Here's how the part is built. I have some questions about the finished solid (model axes, mm). Face numbers are marked on the shaded views. A direction names the side the tool comes from. Give positions to 0.01 mm unless a question says otherwise; leave off trailing zeros. Order: outer loops, then holes, each group sorted by start corner. A loop starts at its lowest first (then second) coordinate and runs counter-clockwise, first axis right, second up.
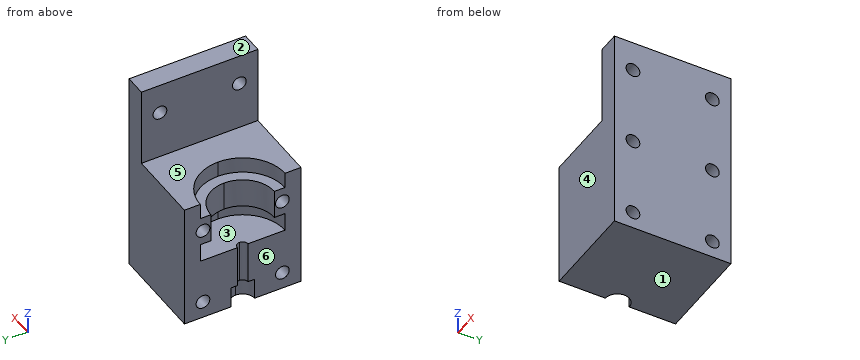
from build123d import *

# Parameters (mm, degrees)
F2_DEPTH  = 24
F1_W      = 3
F1_H      = 22
F3_DEPTH  = 24
F1_W_2    = 4
F4_DEPTH  = 39
F5_DEPTH  = 21
F6_DEPTH  = 15.5
F7_DEPTH  = 12
F8_DEPTH  = 4
F9_R      = 1.3
F10_DEPTH = 18.001


with BuildPart() as f2:
    # F1 (on Top) → F2 (new body)
    with BuildSketch(Plane.XY):
        with BuildLine():
            Line((11, 11), (0, 11))
            Line((0, 11), (0, 8))
            ThreePointArc((0, 8), (5.6568542495, 5.6568542495), (8, 0))
            ThreePointArc((8, 0), (5.6568542495, -5.6568542495), (0, -8))
            Line((0, -8), (0, -11))
            Line((0, -11), (11, -11))
            Line((11, -11), (11, 11))
        make_face()
    extrude(amount=F2_DEPTH)

    # F1 (on Top) → F3 (join)
    with BuildSketch(Plane.XY):
        with Locations((12.5, 0)):
            Rectangle(F1_W, F1_H)
    extrude(amount=F3_DEPTH)

    # F1 (on Top) → F4 (join)
    with BuildSketch(Plane.XY):
        with Locations((16, 0)):
            Rectangle(F1_W_2, F1_H)
    extrude(amount=F4_DEPTH)

    # F1 (on Top) → F5 (join)
    with BuildSketch(Plane.XY):
        with BuildLine():
            ThreePointArc((8, 0), (5.6568542495, 5.6568542495), (0, 8))
            Line((0, 8), (0, 6))
            ThreePointArc((0, 6), (4.2426406871, 4.2426406871), (6, 0))
            ThreePointArc((6, 0), (4.2426406871, -4.2426406871), (0, -6))
            Line((0, -6), (0, -8))
            ThreePointArc((0, -8), (5.6568542495, -5.6568542495), (8, 0))
        make_face()
    extrude(amount=F5_DEPTH)

    # F1 (on Top) → F6 (cut)
    with BuildSketch(Plane.XY):
        with BuildLine():
            ThreePointArc((8, 0), (5.6568542495, 5.6568542495), (0, 8))
            Line((0, 8), (0, 6))
            ThreePointArc((0, 6), (4.2426406871, 4.2426406871), (6, 0))
            ThreePointArc((6, 0), (4.2426406871, -4.2426406871), (0, -6))
            Line((0, -6), (0, -8))
            ThreePointArc((0, -8), (5.6568542495, -5.6568542495), (8, 0))
        make_face()
        with BuildLine():
            Line((0, 6), (0, 8))
            ThreePointArc((0, 8), (-8, 0), (0, -8))
            Line((0, -8), (0, -6))
            ThreePointArc((0, -6), (-6, 0), (0, 6))
        make_face()
    extrude(amount=F6_DEPTH, mode=Mode.SUBTRACT)

    # F1 (on Top) → F7 (join)
    with BuildSketch(Plane.XY):
        with BuildLine():
            ThreePointArc((8, 0), (5.6568542495, 5.6568542495), (0, 8))
            Line((0, 8), (0, 6))
            ThreePointArc((0, 6), (4.2426406871, 4.2426406871), (6, 0))
            ThreePointArc((6, 0), (4.2426406871, -4.2426406871), (0, -6))
            Line((0, -6), (0, -8))
            ThreePointArc((0, -8), (5.6568542495, -5.6568542495), (8, 0))
        make_face()
        with BuildLine():
            ThreePointArc((6, 0), (4.2426406871, 4.2426406871), (0, 6))
            Line((0, 6), (0, 2.25))
            ThreePointArc((0, 2.25), (1.5909902577, 1.5909902577), (2.25, 0))
            ThreePointArc((2.25, 0), (1.5909902577, -1.5909902577), (0, -2.25))
            Line((0, -2.25), (0, -6))
            ThreePointArc((0, -6), (4.2426406871, -4.2426406871), (6, 0))
        make_face()
        with BuildLine():
            ThreePointArc((2.25, 0), (1.5909902577, 1.5909902577), (0, 2.25))
            Line((0, 2.25), (0, 1))
            ThreePointArc((0, 1), (0.7071067812, 0.7071067812), (1, 0))
            ThreePointArc((1, 0), (0.7071067812, -0.7071067812), (0, -1))
            Line((0, -1), (0, -2.25))
            ThreePointArc((0, -2.25), (1.5909902577, -1.5909902577), (2.25, 0))
        make_face()
    extrude(amount=F7_DEPTH)

    # F1 (on Top) → F8 (cut)
    with BuildSketch(Plane.XY):
        with BuildLine():
            ThreePointArc((2.25, 0), (1.5909902577, 1.5909902577), (0, 2.25))
            Line((0, 2.25), (0, 1))
            ThreePointArc((0, 1), (0.7071067812, 0.7071067812), (1, 0))
            ThreePointArc((1, 0), (0.7071067812, -0.7071067812), (0, -1))
            Line((0, -1), (0, -2.25))
            ThreePointArc((0, -2.25), (1.5909902577, -1.5909902577), (2.25, 0))
        make_face()
        with BuildLine():
            Line((0, 1), (0, 2.25))
            ThreePointArc((0, 2.25), (-2.25, 0), (0, -2.25))
            Line((0, -2.25), (0, -1))
            ThreePointArc((0, -1), (-1, 0), (0, 1))
        make_face()
    extrude(amount=F8_DEPTH, mode=Mode.SUBTRACT)

    # F9 (on face) → F10 (cut, through all)
    with BuildSketch(Plane(origin=(0, 0, 0), x_dir=(0, -1, 0), z_dir=(-1, 0, 0))):
        with Locations((-7.5, 18.25)):
            Circle(F9_R)
        with Locations((7.5, 18.25)):
            Circle(F9_R)
        with Locations((7.5, 3.25)):
            Circle(F9_R)
        with Locations((-7.5, 3.25)):
            Circle(F9_R)
        with Locations((-7.5, 33.25)):
            Circle(F9_R)
        with Locations((7.5, 33.25)):
            Circle(F9_R)
    extrude(amount=-F10_DEPTH, mode=Mode.SUBTRACT)


solid = f2.part
Q1. I need wall thicknesses on L1, parallel to Z at x = 16.15, y = -7.5; L2, parallel to Z at x = 13.5, y = 7.5; L3, parallel to Z at x = 11.5, y = -9.5. Which ranges of each line are inside material? Lowest first, please.
Filled sheet:
L1: z = 0 to 1.95, 4.55 to 16.95, 19.55 to 31.95, 34.55 to 39
L2: z = 0 to 1.95, 4.55 to 16.95, 19.55 to 24
L3: z = 0 to 24
Q2. I'm going to push flat-ended pins straight in: P1, Ø12, axis at y = -4, z = 30.5, coming from the -X side; P2, Ø4, axis at x = 10, y = -5, coming from the +Z side. Where does each tip first touch, or does it pass through?
Filled sheet:
P1: stops at x = 14
P2: stops at z = 24
Q3. Thinking about a two-plate mould opening in Z: for the marked faces 1, 2, 3 and 4, which applies, released by +Z, released by -Z, zero draft, split by the parting line, or undercut?
Filled sheet:
face 1: released by -Z
face 2: released by +Z
face 3: undercut
face 4: zero draft
Q4. If we section it at A-A on z = 33.25: List the corners of the cut face in (x, y) for me.
Filled sheet:
outline: (14, -11) - (18, -11) - (18, -8.8) - (14, -8.8) - close; (14, -6.2) - (18, -6.2) - (18, 6.2) - (14, 6.2) - close; (14, 8.8) - (18, 8.8) - (18, 11) - (14, 11) - close
Q5. If we section it at D-D on z = 12.5: List the corners of the cut face in (x, y) for me, plus the area to 3 significant figures.
Filled sheet:
outline: (0, -11) - (18, -11) - (18, 11) - (0, 11) - (0, 8) arc R8 cw to (0, -8) - close
area: 295 mm2
Q6. If we section it at C-C on x = 4.5: List the corners of the cut face in (y, z) for me, plus the area to 3 significant figures.
Filled sheet:
outline: (-11, 0) - (11, 0) - (11, 24) - (6.61, 24) - (6.61, 21) - (3.97, 21) - (3.97, 15.5) - (6.61, 15.5) - (6.61, 12) - (-6.61, 12) - (-6.61, 15.5) - (-3.97, 15.5) - (-3.97, 21) - (-6.61, 21) - (-6.61, 24) - (-11, 24) - close; hole circle Ø2.6 at (-7.5, 3.25); hole circle Ø2.6 at (-7.5, 18.25); hole circle Ø2.6 at (7.5, 3.25); hole circle Ø2.6 at (7.5, 18.25)
area: 377 mm2
Q7. If we section it at B-B on y = 7.5: List the corners of the cut face in (x, z) for me.
Filled sheet:
outline: (0, 0) - (18, 0) - (18, 1.95) - (0, 1.95) - close; (0, 4.55) - (18, 4.55) - (18, 16.95) - (0, 16.95) - (0, 15.5) - (2.78, 15.5) - (2.78, 12) - (0, 12) - close; (0, 19.55) - (18, 19.55) - (18, 31.95) - (14, 31.95) - (14, 24) - (2.78, 24) - (2.78, 21) - (0, 21) - close; (14, 34.55) - (18, 34.55) - (18, 39) - (14, 39) - close
Q8. For the marked faces 5 and 6, which set-ups out of +Z, -Z, +X, -X, +Y, -Y let a thin tool reach every point of the face, with its end or its side?
Filled sheet:
face 5: +Z, -X, +Y, -Y
face 6: +Z, -Z, -X, +Y, -Y
